Build history of the part. All positions in model axes, mm. Face numbers are marked on the shaded views. A direction names the side the tool comes from. Round coordinates to 2 decimals unless told otherwise and drop trailing zeros. Write each loop counter-clockwise with the first axis right and the second up, starting at its lowest first coordinate (ties: lowest second). Pieces come first, ordered by that corner, then holes.
Item 1: Mould opens along X. For the marked faces 1, 2 and 3 say: +X half, -X half, draft (parallel to the pull), parting line (faces both ways), or undercut.
Item 2: Band-saw the part on B-B, the plane z = -27.5. Write the cut outline in (x, y).
Item 3: Drop flat-ended pins along their axis: pin 1 Ø6.5 at (y, z) = (-7.5, -8.5) entering from +X; pin 2 Ø5.5 at (x, y) = (15.5, 15.5) entering from -Z; pin 3 Ø8 at (x, z) = (15.5, -35.5) entering from -Y; pin 4 Ø6 at (x, z) = (14.5, -10.5) entering from +Y. Give the stop position or say it passes through.
Item 4: Band-saw the part on A-A, the plane y = -15.5. Write the cut outline in (x, z).
Item 5: 3-axis set-ups, long thin cutter, end or side, ignore diameter. For the marked faces 4 and 5: which of +Z, -Z, +X, -X, +Y, -Y reach the whole face in a straight line?
Item 6: Wall check: probe 1 along X at (y, z) = (4, 2); probe 2 along Y at (x, z) = (15.5, 1.25); probe 3 along Y at (x, z) = (0, 1). Give the ranges that are in metal, low to high.
Item 7: Band-saw the part on D-D, the plane y = -5. Write the cut outline in (x, z) (3 decimals).
Item 8: Band-saw the part on C-C, the plane x = 15.5. Write the cut outline in (y, z), then the cut area to 3 significant figures.
```python
from build123d import *

# Parameters (mm, degrees)
SKETCH_1_W          = 50
SKETCH_1_H          = 51
SKETCH_1_R          = 11
SKETCH_1_R_2        = 1.75
EXTRUDE_1_DEPTH     = 3
CHAMFER_1_SIZE      = 5
SKETCH_2_W          = 50
SKETCH_2_H          = 3
EXTRUDE_2_DEPTH     = 50
CHAMFER_2_SIZE      = 5
CUT_EXTRUDE_1_DEPTH = 50
EXTRUDE_3_DEPTH     = 3
EXTRUDE_4_DEPTH     = 3


with BuildPart() as part:
    # 草图1 → 凸台-拉伸1 (new body)
    with BuildSketch(Plane.XY):
        Rectangle(SKETCH_1_W, SKETCH_1_H)
        with Locations((0, 4.5)):
            Circle(SKETCH_1_R, mode=Mode.SUBTRACT)
        with Locations((-15.5, 15.5)):
            Circle(SKETCH_1_R_2, mode=Mode.SUBTRACT)
        with Locations(Location((-15.5, -15.5, 0), (0, 0, 180))):
            Circle(SKETCH_1_R_2, mode=Mode.SUBTRACT)
        with Locations((15.5, -15.5)):
            Circle(SKETCH_1_R_2, mode=Mode.SUBTRACT)
        with Locations(Location((15.5, 15.5, 0), (0, 0, 180))):
            Circle(SKETCH_1_R_2, mode=Mode.SUBTRACT)
    extrude(amount=EXTRUDE_1_DEPTH)

    # 倒角1
    chamfer_1_edges = [part.edges().sort_by_distance(p)[0] for p in [
        (-25, 25.5, 1.5),
        (25, 25.5, 1.5),
    ]]
    chamfer(chamfer_1_edges, length=CHAMFER_1_SIZE)

    # 草图2 → 凸台-拉伸2 (add)
    with BuildSketch(Plane(origin=(0, 0, 0), x_dir=(-1, 0, 0), z_dir=(0, 0, -1))):
        with Locations((0, -24)):
            Rectangle(SKETCH_2_W, SKETCH_2_H)
    extrude(amount=EXTRUDE_2_DEPTH)

    # 倒角2
    chamfer_2_edges = [part.edges().sort_by_distance(p)[0] for p in [
        (-25, -24, -50),
        (25, -24, -50),
    ]]
    chamfer(chamfer_2_edges, length=CHAMFER_2_SIZE)

    # 草图3 → 切除-拉伸1 (cut)
    with BuildSketch(Plane(origin=(0, -22.5, 0), x_dir=(1, 0, 0), z_dir=(0, 1, 0))):
        with BuildLine():
            Line((-17.1, 39), (-17.1, 9))
            ThreePointArc((-17.1, 9), (-15, 6.9), (-12.9, 9))
            Line((-12.9, 9), (-12.9, 39))
            ThreePointArc((-12.9, 39), (-15, 41.1), (-17.1, 39))
        make_face()
        with BuildLine():
            Line((12.9, 39), (12.9, 9))
            ThreePointArc((12.9, 9), (15, 6.9), (17.1, 9))
            Line((17.1, 9), (17.1, 39))
            ThreePointArc((17.1, 39), (15, 41.1), (12.9, 39))
        make_face()
    extrude(amount=-CUT_EXTRUDE_1_DEPTH, mode=Mode.SUBTRACT)

    # 草图4 → 凸台-拉伸3 (add)
    with BuildSketch(Plane(origin=(25, 0, 0), x_dir=(0, 0, -1), z_dir=(1, 0, 0))):
        Polygon((0, -2.5), (13, -22.5), (0, -22.5), align=None)
    extrude(amount=-EXTRUDE_3_DEPTH)

    # 草图5 → 凸台-拉伸4 (add)
    with BuildSketch(Plane.ZY.offset(25)):
        Polygon((0, -22.5), (0, -2.5), (-13, -22.5), align=None)
    extrude(amount=-EXTRUDE_4_DEPTH)


solid = part.part
```
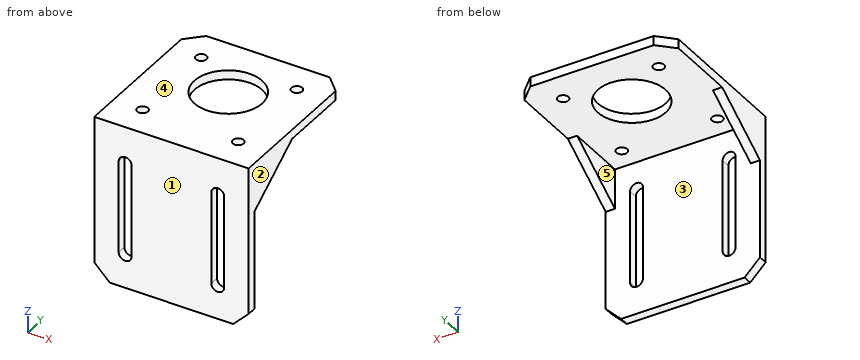
Results:
1. face 1: draft
1. face 2: +X half
1. face 3: undercut
2. outline: (-25, -25.5) - (-17.1, -25.5) - (-17.1, -22.5) - (-25, -22.5) - close; (-12.9, -25.5) - (12.9, -25.5) - (12.9, -22.5) - (-12.9, -22.5) - close; (17.1, -25.5) - (25, -25.5) - (25, -22.5) - (17.1, -22.5) - close
3. pin 1: passes through
3. pin 2: stops at z = 0
3. pin 3: stops at y = -25.5
3. pin 4: stops at y = -22.5
4. outline: (-25, -8.45) - (-22, -8.45) - (-22, 0) - (-17.25, 0) - (-17.25, 3) - (-25, 3) - close; (-13.75, 0) - (13.75, 0) - (13.75, 3) - (-13.75, 3) - close; (17.25, 0) - (22, 0) - (22, -8.45) - (25, -8.45) - (25, 3) - (17.25, 3) - close
5. face 4: +Z, +X, -X, +Y, -Y
5. face 5: -Z, +Y
6. probe 1: x = -25 to -10.99, 10.99 to 25
6. probe 2: y = -25.5 to -17.25, -13.75 to 13.75, 17.25 to 25.5
6. probe 3: y = -25.5 to -6.5, 15.5 to 25.5
7. outline: (-25, -1.625) - (-22, -1.625) - (-22, 0) - (-5.545, 0) - (-5.545, 3) - (-25, 3) - close; (5.545, 0) - (22, 0) - (22, -1.625) - (25, -1.625) - (25, 3) - (5.545, 3) - close
8. outline: (-25.5, -50) - (-22.5, -50) - (-22.5, -41.04) - (-25.5, -41.04) - close; (-25.5, -6.96) - (-22.5, -6.96) - (-22.5, 0) - (-17.25, 0) - (-17.25, 3) - (-25.5, 3) - close; (-13.75, 0) - (13.75, 0) - (13.75, 3) - (-13.75, 3) - close; (17.25, 0) - (25.5, 0) - (25.5, 3) - (17.25, 3) - close
8. area: 180 mm2
